from build123d import *

# Parameters (mm, degrees)
F0_W     = 65.532
F0_H     = 86.995
F1_DEPTH = 41.275
F2_R     = 5.3975
F3_DEPTH = 38.1
F4_R     = 6.35


with BuildPart() as f1:
    # F0 (on Top) → F1 (new body)
    with BuildSketch(Plane.XY):
        Rectangle(F0_W, F0_H)
    extrude(amount=F1_DEPTH)

    # F2 (on face) → F3 (cut)
    with BuildSketch(Plane.XY.offset(41.275)):
        with Locations((-24.1935, 34.925)):
            Circle(F2_R)
        with Locations((-24.1935, 20.955)):
            Circle(F2_R)
        with Locations((-24.1935, 6.985)):
            Circle(F2_R)
        with Locations((-24.1935, -6.985)):
            Circle(F2_R)
        with Locations((-24.1935, -20.955)):
            Circle(F2_R)
        with Locations((-24.1935, -34.925)):
            Circle(F2_R)
        with Locations((-12.095125, 27.94)):
            Circle(F2_R)
        with Locations((-12.095125, 13.97)):
            Circle(F2_R)
        with Locations((-12.095125, 0)):
            Circle(F2_R)
        with Locations((-12.095125, -13.97)):
            Circle(F2_R)
        with Locations((-12.095125, -27.94)):
            Circle(F2_R)
        with Locations((12.101625, 0)):
            Circle(F2_R)
        with Locations((12.101625, 13.97)):
            Circle(F2_R)
        with Locations((12.101625, -13.97)):
            Circle(F2_R)
        with Locations((0.00325, 6.985)):
            Circle(F2_R)
        with Locations((0.00325, 20.955)):
            Circle(F2_R)
        with Locations((0.00325, 34.925)):
            Circle(F2_R)
        with Locations((12.101625, -27.94)):
            Circle(F2_R)
        with Locations((12.101625, 27.94)):
            Circle(F2_R)
        with Locations((0.00325, -6.985)):
            Circle(F2_R)
        with Locations((0.00325, -20.955)):
            Circle(F2_R)
        with Locations((0.00325, -34.925)):
            Circle(F2_R)
        with Locations((24.2, 6.985)):
            Circle(F2_R)
        with Locations((24.2, 20.955)):
            Circle(F2_R)
        with Locations((24.2, 34.925)):
            Circle(F2_R)
        with Locations((24.2, -6.985)):
            Circle(F2_R)
        with Locations((24.2, -20.955)):
            Circle(F2_R)
        with Locations((24.2, -34.925)):
            Circle(F2_R)
    extrude(amount=-F3_DEPTH, mode=Mode.SUBTRACT)

    # F4
    f4_edges = [f1.edges().sort_by_distance(p)[0] for p in [
        (-32.766, -43.4975, 20.6375),
        (32.766, -43.4975, 20.6375),
        (32.766, 43.4975, 20.6375),
        (-32.766, 43.4975, 20.6375),
    ]]
    fillet(f4_edges, radius=F4_R)


solid = f1.part
The model under review builds one solid part; all positions refer to its coordinate system, in mm. A direction names the side the tool comes from. Round coordinates to 2 decimals unless told otherwise and drop trailing zeros. Order: outer loops, then holes, each group sorted by start corner. A loop starts at its lowest first (then second) coordinate and runs counter-clockwise, first axis right, second up. Notation, with made-up numbers: (24.25, -12) -> (42.25, -12) arc R16 cw to (42.25, 15) -> close; hole circle Ø9 at (52.25, 79). An arc over 180 degrees is marked (long way). Write item = value, one per line. Start each with the question number.
Item 1: Clearance check with a flat-ended pin moving along its axis: pin 1 Ø3 at (x, y) = (23.5, 5.5) entering from +Z (3 decimals). State where the tip first meets the part, or that it passes through.
Item 2: Consider section D-D on x = 1.5. Write out the cut boundary in (y, z) (1 decimal).
Item 3: Mouldability with a two-part tool opening along Y and no side actions: class faces 1 (the face through (0, 1, 41.275)), 2 (the face through (0, 35, 3.175)), 3 (the face through (30.856, 41.687, 20.926)) as released by +Y, released by -Y, zero draft, split by the parting line, or undercut.
Item 4: For faces 4 (the face through (12, -14, 3.175)), 5 (the face through (0, -43.498, 20)), list the 3-axis set-ups (+Z, -Z, +X, -X, +Y, -Y) from which the entire face can be reached by the end or side of a thin tool; tool diameter is ignored.
Item 5: Consider section B-B on x = 24.2. Write out the cut boundary in (y, z) (1 decimal).
Item 6: Consider section C-C on z = 16. Count the separate pieces of the cut face and the enclosed holes in it, plus the area to 3 significant figures.
Item 7: Consider section A-A on y = -13.97. Write out the cut boundary in (x, z) (3 decimals), plus the area to 3 significant figures.
Item 8: For line 1 along X through (y, z) = (15, 33); line 2 along X through (y, z) = (31, 4); line 3 along X through (y, z) = (-37, 31), list the stretches that pass through material, from the lowest coordinate up.
Conclusion:
q1.pin_1 = 3.175
q2.outline = (-43.5, 0) -> (43.5, 0) -> (43.5, 41.3) -> (40.1, 41.3) -> (40.1, 3.2) -> (29.7, 3.2) -> (29.7, 41.3) -> (26.1, 41.3) -> (26.1, 3.2) -> (15.8, 3.2) -> (15.8, 41.3) -> (12.2, 41.3) -> (12.2, 3.2) -> (1.8, 3.2) -> (1.8, 41.3) -> (-1.8, 41.3) -> (-1.8, 3.2) -> (-12.2, 3.2) -> (-12.2, 41.3) -> (-15.8, 41.3) -> (-15.8, 3.2) -> (-26.1, 3.2) -> (-26.1, 41.3) -> (-29.7, 41.3) -> (-29.7, 3.2) -> (-40.1, 3.2) -> (-40.1, 41.3) -> (-43.5, 41.3) -> close
q3.face_1 = zero draft
q3.face_2 = undercut
q3.face_3 = released by +Y
q4.face_4 = +Z
q4.face_5 = +Z, -Z, +X, -X, -Y
q5.outline = (-43.5, 0) -> (43.5, 0) -> (43.5, 41.3) -> (40.3, 41.3) -> (40.3, 3.2) -> (29.5, 3.2) -> (29.5, 41.3) -> (26.4, 41.3) -> (26.4, 3.2) -> (15.6, 3.2) -> (15.6, 41.3) -> (12.4, 41.3) -> (12.4, 3.2) -> (1.6, 3.2) -> (1.6, 41.3) -> (-1.6, 41.3) -> (-1.6, 3.2) -> (-12.4, 3.2) -> (-12.4, 41.3) -> (-15.6, 41.3) -> (-15.6, 3.2) -> (-26.4, 3.2) -> (-26.4, 41.3) -> (-29.5, 41.3) -> (-29.5, 3.2) -> (-40.3, 3.2) -> (-40.3, 41.3) -> (-43.5, 41.3) -> close
q6.separate_pieces = 1
q6.enclosed_holes = 28
q6.area = 3,100 mm2
q7.outline = (-32.766, 0) -> (32.766, 0) -> (32.766, 41.275) -> (17.499, 41.275) -> (17.499, 3.175) -> (6.704, 3.175) -> (6.704, 41.275) -> (-6.698, 41.275) -> (-6.698, 3.175) -> (-17.493, 3.175) -> (-17.493, 41.275) -> (-32.766, 41.275) -> close
q7.area = 1,880 mm2
q8.line_1 = -32.77 to -17.39, -6.8 to 6.8, 17.4 to 32.77
q8.line_2 = -32.77 to -27.9, -20.49 to -16.54, -7.65 to -3.7, 3.71 to 7.66, 16.55 to 20.49, 27.91 to 32.77
q8.line_3 = -32.77 to -29.18, -19.21 to -4.98, 4.99 to 19.22, 29.18 to 32.77
